```python
from build123d import *

# Parameters (mm, degrees)
BOSS_EXTRUDE1_DEPTH = 50
SKETCH3_W           = 40
SKETCH3_H           = 50
CUT_EXTRUDE1_DEPTH  = 5
SKETCH7_W           = 40
SKETCH7_H           = 50
CUT_EXTRUDE2_DEPTH  = 5
FILLET1_R           = 10


# Read off the part's stored shape, not the designer's step: M5 Clearance Hole1, M5 Clearance Hole2
with BuildPart() as part:
    # Sketch1 → Boss-Extrude1 (new body)
    with BuildSketch(Plane(origin=(0, 0, 0), x_dir=(1, 0, 0), z_dir=(0, 1, 0))):
        Polygon((10, 10), (10, 80), (0, 80), (0, 0), (180, 0), (180, 10), align=None)
        Polygon((39.142135624, 10), (10, 39.142135624), (10, 25), (25, 10), align=None)
    extrude(amount=BOSS_EXTRUDE1_DEPTH)

    # Sketch3 → Cut-Extrude1 (cut)
    with BuildSketch(Plane.XY.offset(-10)):
        with Locations((160, 25)):
            Rectangle(SKETCH3_W, SKETCH3_H)
    extrude(amount=CUT_EXTRUDE1_DEPTH, mode=Mode.SUBTRACT)

    # M5 Clearance Hole1 outline → M5 Clearance Hole1 (revolve, cut)
    with BuildSketch(Plane(origin=(170, 40, 0), x_dir=(1, 0, 0), z_dir=(0, -1, 0))):
        Polygon((2.75, -4.975), (2.75, 0), (0, 0), (0, -5), (2.775, -5), align=None)
    revolve(axis=Axis((170, 40, 0), (0, 0, 1)), mode=Mode.SUBTRACT)

    # M5 Clearance Hole1 2 outline → M5 Clearance Hole1 2 (revolve, cut)
    with BuildSketch(Plane(origin=(150, 40, 0), x_dir=(1, 0, 0), z_dir=(0, -1, 0))):
        Polygon((2.75, -4.975), (2.75, 0), (0, 0), (0, -5), (2.775, -5), align=None)
    revolve(axis=Axis((150, 40, 0), (0, 0, 1)), mode=Mode.SUBTRACT)

    # M5 Clearance Hole1 3 outline → M5 Clearance Hole1 3 (revolve, cut)
    with BuildSketch(Plane(origin=(150, 10, 0), x_dir=(1, 0, 0), z_dir=(0, -1, 0))):
        Polygon((2.75, -4.975), (2.75, 0), (0, 0), (0, -5), (2.775, -5), align=None)
    revolve(axis=Axis((150, 10, 0), (0, 0, 1)), mode=Mode.SUBTRACT)

    # M5 Clearance Hole1 4 outline → M5 Clearance Hole1 4 (revolve, cut)
    with BuildSketch(Plane(origin=(170, 10, 0), x_dir=(1, 0, 0), z_dir=(0, -1, 0))):
        Polygon((2.75, -4.975), (2.75, 0), (0, 0), (0, -5), (2.775, -5), align=None)
    revolve(axis=Axis((170, 10, 0), (0, 0, 1)), mode=Mode.SUBTRACT)

    # Sketch7 → Cut-Extrude2 (cut)
    with BuildSketch(Plane.ZY):
        with Locations((-60, 25)):
            Rectangle(SKETCH7_W, SKETCH7_H)
    extrude(amount=-CUT_EXTRUDE2_DEPTH, mode=Mode.SUBTRACT)

    # M5 Clearance Hole2 outline → M5 Clearance Hole2 (revolve, cut)
    with BuildSketch(Plane(origin=(0, 40, -70), x_dir=(0, 1, 0), z_dir=(0, 0, -1))):
        Polygon((2.75, 5.025), (2.75, 10), (0, 10), (0, 5), (2.775, 5), align=None)
    revolve(axis=Axis((0, 40, -70), (1, 0, 0)), mode=Mode.SUBTRACT)

    # M5 Clearance Hole2 2 outline → M5 Clearance Hole2 2 (revolve, cut)
    with BuildSketch(Plane(origin=(0, 10, -70), x_dir=(0, 1, 0), z_dir=(0, 0, -1))):
        Polygon((2.75, 5.025), (2.75, 10), (0, 10), (0, 5), (2.775, 5), align=None)
    revolve(axis=Axis((0, 10, -70), (1, 0, 0)), mode=Mode.SUBTRACT)

    # M5 Clearance Hole2 3 outline → M5 Clearance Hole2 3 (revolve, cut)
    with BuildSketch(Plane(origin=(0, 40, -50), x_dir=(0, 1, 0), z_dir=(0, 0, -1))):
        Polygon((2.75, 5.025), (2.75, 10), (0, 10), (0, 5), (2.775, 5), align=None)
    revolve(axis=Axis((0, 40, -50), (1, 0, 0)), mode=Mode.SUBTRACT)

    # M5 Clearance Hole2 4 outline → M5 Clearance Hole2 4 (revolve, cut)
    with BuildSketch(Plane(origin=(0, 10, -50), x_dir=(0, 1, 0), z_dir=(0, 0, -1))):
        Polygon((2.75, 5.025), (2.75, 10), (0, 10), (0, 5), (2.775, 5), align=None)
    revolve(axis=Axis((0, 10, -50), (1, 0, 0)), mode=Mode.SUBTRACT)

    # Fillet1
    fillet1_edges = [part.edges().sort_by_distance(p)[0] for p in [
        (0, 25, 0),
    ]]
    fillet(fillet1_edges, radius=FILLET1_R)


solid = part.part
```
Work out the finished part from the listing and answer in its coordinate system (mm). A direction names the side the tool comes from. Give positions to 0.01 mm unless a question says otherwise; leave off trailing zeros. Order: outer loops, then holes, each group sorted by start corner. A loop starts at its lowest first (then second) coordinate and runs counter-clockwise, first axis right, second up.
1. Section B-B, the plane y = 25 is taken. Determine the outline of the cut face in (x, z).
Result sheet:
outline: (0, -40) - (5, -40) - (5, -80) - (10, -80) - (10, -39.14) - (39.14, -10) - (140, -10) - (140, -5) - (180, -5) - (180, 0) - (10, 0) arc R10 ccw to (0, -10) - close; hole (10, -25) - (25, -10) - (10, -10) - close
2. Section A-A, the plane z = -70 is taken. Determine the outline of the cut face in (x, y) (3 decimals), and give its area (3 significant figures).
Result sheet:
outline: (5, 0) - (10, 0) - (10, 7.25) - (5.025, 7.25) - (5, 7.225) - close; (5, 12.775) - (5.025, 12.75) - (10, 12.75) - (10, 37.25) - (5.025, 37.25) - (5, 37.225) - close; (5, 42.775) - (5.025, 42.75) - (10, 42.75) - (10, 50) - (5, 50) - close
area: 195 mm2
3. Each of these flat-tipped pins is pushed along its axis until it touches: P1, Ø6.5, axis at y = 40, z = -50, coming from the +X side; P2, Ø6.5, axis at x = 170, y = 10, coming from the -Z side; P3, Ø3.5, axis at x = 170, y = 40, coming from the +Z side; P4, Ø1.5, axis at y = 25.5, z = -7.5, coming from the +X side. Where does it stop, or does it pass through?
Result sheet:
P1: stops at x = 10
P2: stops at z = -5
P3: passes through
P4: stops at x = 140
4. The mould has two halves that part along Y. Classify faces 1 (the cylindrical face through (7.547, 9.642, -47.273)), 2 (the flat face through (56, 50, -8)), 3 (the flat face through (160, 25, -5)): released by +Y, released by -Y, zero draft, split by the parting line, or undercut.
Result sheet:
face 1: undercut
face 2: released by +Y
face 3: zero draft
5. Section C-C, the plane x = 170 is taken. Determine the outline of the cut face in (y, z) (3 decimals).
Result sheet:
outline: (0, -5) - (7.225, -5) - (7.25, -4.975) - (7.25, 0) - (0, 0) - close; (12.75, -4.975) - (12.775, -5) - (37.225, -5) - (37.25, -4.975) - (37.25, 0) - (12.75, 0) - close; (42.75, -4.975) - (42.775, -5) - (50, -5) - (50, 0) - (42.75, 0) - close
6. For faces 4 (the flat face through (18, 25, -10)), 5 (the flat face through (5, 25, -60)), 6 (the flat face through (140, 25, -8)), determine the directions among +Z, -Z, +X, -X, +Y, -Y from which every point of the face is accessible in a straight line to the end or side of a thin tool.
Result sheet:
face 4: +Y, -Y
face 5: -Z, -X, +Y, -Y
face 6: -Z, +X, +Y, -Y
7. Straight lines are drawn through the part: L1, parallel to Y at x = 150, z = -1.9; L2, parallel to X at y = 21, z = -55; L3, parallel to Z at x = 90.5, y = 11. For each, find the intervals that lie inside material, in ascending order.
Result sheet:
L1: y = 0 to 7.25, 12.75 to 37.25, 42.75 to 50
L2: x = 5 to 10
L3: z = -10 to 0
8. Section D-D, the plane y = 10 is taken. Give the number of separate pieces and of enclosed holes in the cut face, and give its area (3 significant figures).
Result sheet:
separate pieces: 5
enclosed holes: 1
area: 2,280 mm2
